Here's how the part is built. I have some questions about the finished solid (model axes, mm). A direction names the side the tool comes from. Round coordinates to 2 decimals unless told otherwise and drop trailing zeros. Loops run counter-clockwise (first coordinate to the right, second up) from the corner with the lowest first, then second, coordinate; pieces in that order, holes last. Notation, with made-up numbers: M -30.5,29.25 L 20.5,29.25 A24 ccw 20.5,50.25 Z; hole C -6.75,-15.5 d10. An arc over 180 degrees is marked long. Use a Markdown table: item, result.
Autodesk Inventor part; units mm, degrees
ref_plane "YZ Plane" through (0, 0, 0) normal (1, 0, 0) x (0, 1, 0)
ref_plane "XZ Plane" through (0, 0, 0) normal (0, 1, 0) x (-1, 0, 0)
ref_plane "XY Plane" through (0, 0, 0) normal (0, 0, 1) x (1, 0, 0)
sketch "Sketch1" plane through (0, 0, 0) normal (0, 1, 0) x (-1, 0, 0)
  circle A0 centre (0, 0) radius 4
  circle A1 centre (0, 0) radius 5.5
  circle A2 centre (0, 0) radius 22.5
  line L0 (0, 0) -> (-19.5, 0) construction
  dimension "d0" = 8
  dimension "d1" = 11
  dimension "d2" = 45
  dimension "d3" = 19.5
extrude "Extrusion1" add sketch "Sketch1" along normal blind 2.2 contours A0 | A1 | A2
extrude "Extrusion2" add sketch "Sketch1" against normal blind 3.8 contours A0
extrude "Extrusion3" add sketch "Sketch1" against normal blind 1.5 contours A1
hole "Hole1" at (19.5, 0, 0) direction (0, 1, 0) diameter 2 end through all
hole "Hole2" at (0, -3.8, 0) direction (0, 1, 0) diameter 3 end through all
hole "Hole3" at (0, -3.8, 0) direction (0, 1, 0) diameter 6 depth 4
hole "Hole4" at (0, 2.2, 0) direction (0, -1, 0) diameter 6 depth 1
pattern_circular "Circular Pattern1" count 8 over 360 about axis through (0, -10, 0) along (0, 1, 0) of "Hole1"
properties part number "servo arm TGY-S4505B round large"
1. Imagine slicing it at A-A, the plane x = 0. State how many separate pieces and enclosed holes the cut face has, then the cut area to 3 significant figures.
Answer sheet:
| item | result |
|---|---|
| separate pieces | 4 |
| enclosed holes | 0 |
| area | 92.1 mm2 |
2. For pin 1 Ø2.5 at (x, z) = (-13.79, 13.79) entering from -Y; pin 2 Ø2 at (x, y) = (-15, 1.5) entering from -Z; pin 3 Ø1 at (x, y) = (-8.5, 1.5) entering from +Z, each with a flat end and sliding along its axis, tell me the tip position at first contact or that it passes through.
Answer sheet:
| item | result |
|---|---|
| pin 1 | y = 0 |
| pin 2 | z = -17.61 |
| pin 3 | z = 21.03 |
3. We'd pull the mould along Z, two halves only. Please class faces 4 (the face through (0.867, -2.634, -3.905)), 5 (the face through (-0.217, 1.115, 20.476)), 6 (the face through (-1, -3.8, 3)): +Z half, -Z half, draft (parallel to the pull), parting line (faces both ways), or undercut.
Answer sheet:
| item | result |
|---|---|
| face 4 | parting line |
| face 5 | undercut |
| face 6 | draft |
4. Imagine slicing it at C-C, the plane x = -19.5. Write out the boundary of the cut face in (y, z).
Answer sheet:
| item | result |
|---|---|
| outline | M 0,-11.22 L 2.2,-11.22 L 2.2,-1 L 0,-1 Z; M 0,1 L 2.2,1 L 2.2,11.22 L 0,11.22 Z |
5. I need wall thicknesses on probe 1 along Y at (x, z) = (8.5, 3.5); probe 2 along X at (y, z) = (0.5, 19.5); probe 3 along Y at (x, z) = (-4, 1). Which ranges of each line are inside material? Lowest first, please. Write a range as from..to.
Answer sheet:
| item | result |
|---|---|
| probe 1 | 0..2.2 |
| probe 2 | -11.22..-1, 1..11.22 |
| probe 3 | -1.5..2.2 |
6. Which directions (+Z, -Z, +X, -X, +Y, -Y) give clear straight access to the entire face, cutting with the end or side of a thin tool? Please do faces 1 (the face through (0, -2, 3)), 2 (the face through (1.3, 1.2, 1.3)), 3 (the face through (0.217, 1.115, -20.476)).
Answer sheet:
| item | result |
|---|---|
| face 1 | -Y |
| face 2 | +Y |
| face 3 | +Y, -Y |
7. Imagine slicing it at D-D, the plane y = -2.85. Write out the boundary of the cut face in (x, z).
Answer sheet:
| item | result |
|---|---|
| outline | C 0,0 d8; hole C 0,0 d6 |
